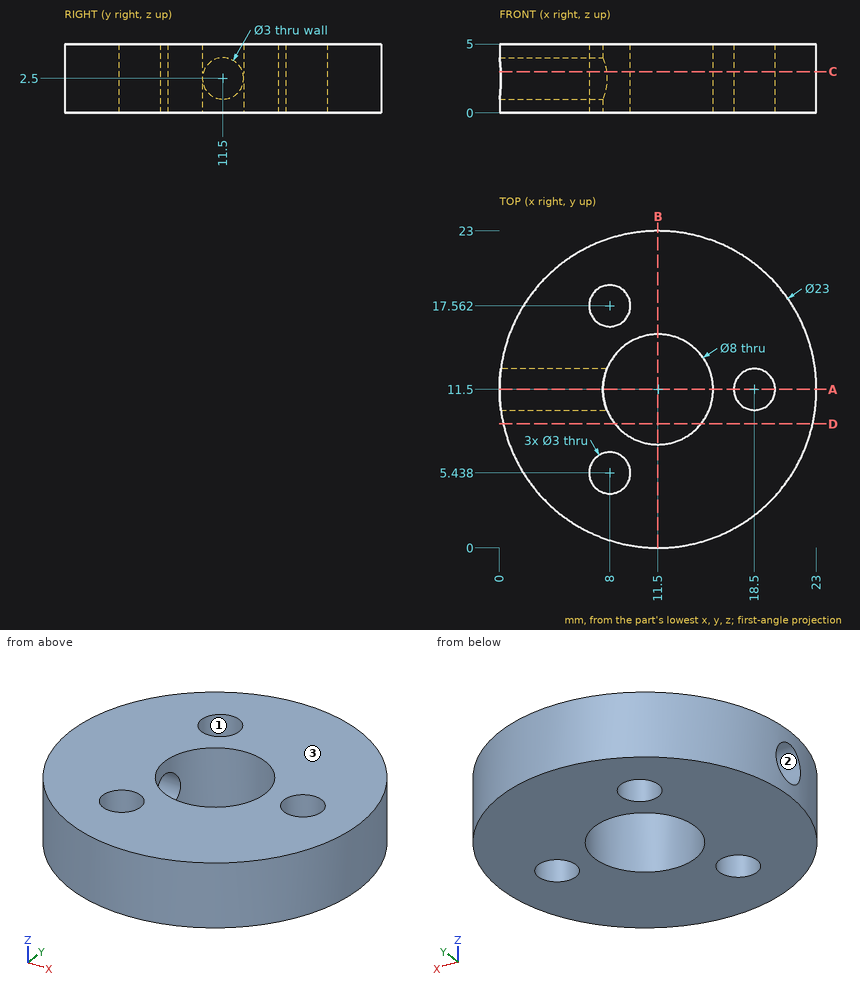
Input: dimensioned drawing with shaded views. Units: mm. Origin: part minimum x, y, z. Round coordinates to 2 decimals unless told otherwise and drop trailing zeros. Loops run counter-clockwise (first coordinate to the right, second up) from the corner with the lowest first, then second, coordinate; pieces in that order, holes last. Notation, with made-up numbers: M 68,-19 L 80,-19 A4 ccw 80,-12 Z; hole C 20,71.25 d8. An arc over 180 degrees is marked long. Answer in a Markdown table with one row per item. Add a question column.
1. Section C-C (z = 3). Output: boundary loops of the cut face in (x, y), and give its area (3 significant figures).
2. Mould query, pull axis Z, two halves, no side actions, for the marked faces 1, 2 and 3. Classes: released by +Z, released by -Z, zero draft, split by the parting line, or undercut.
3. Contact query for flat-ended pins moving along their axis: pin 1 (8 mm diameter, centred on x = 9, y = 9.5, fed in from -Z); pin 2 (1 mm diameter, centred on x = 4.5, z = 4, fed in from -Y); pin 3 (1 mm diameter, centred on x = 13, z = 1.5, fed in from -Y). Output: stop coordinate, or through.
4. Section A-A (y = 11.5). Output: boundary loops of the cut face in (x, z), and give its area (3 significant figures).
5. Ray query, probe 1 along Y at (x, z) = (8, 3.2) (1 decimal); probe 2 along Y at (x, z) = (11.5, 4.55); probe 3 along Y at (x, z) = (19, 2.5) (1 decimal). Return the intervals inside material, ascending.
6. Section D-D (y = 9). Output: boundary loops of the cut face in (x, z) (1 decimal).
7. Section B-B (x = 11.5). Output: boundary loops of the cut face in (y, z), and give its area (3 significant figures).
Values follow:
| question | item | result |
|---|---|---|
| 1 | outline | M 0.09,10.09 A11.5 ccw long 0.09,12.91 L 7.76,12.91 A4 cw long 7.76,10.09 Z; hole C 8,5.44 d3; hole C 8,17.56 d3; hole C 18.5,11.5 d3 |
| 1 | area | 323 mm^2 |
| 2 | face 1 | zero draft |
| 2 | face 2 | undercut |
| 2 | face 3 | released by +Z |
| 3 | pin 1 | z = 0 |
| 3 | pin 2 | y = 2.01 |
| 3 | pin 3 | y = 0.04 |
| 4 | outline | M 0,0 L 7.5,0 L 7.5,1 L 0,1 Z; M 0,4 L 7.5,4 L 7.5,5 L 0,5 Z; M 15.5,0 L 17,0 L 17,5 L 15.5,5 Z; M 20,0 L 23,0 L 23,5 L 20,5 Z |
| 4 | area | 37.5 mm^2 |
| 5 | probe 1 | 0.5 to 3.9, 6.9 to 9.6, 13.4 to 16.1, 19.1 to 22.5 |
| 5 | probe 2 | 0 to 7.5, 15.5 to 23 |
| 5 | probe 3 | 2.8 to 10.1, 12.9 to 20.2 |
| 6 | outline | M 0.3,0 L 8.4,0 L 8.4,5 L 0.3,5 Z; M 14.6,0 L 22.7,0 L 22.7,5 L 14.6,5 Z |
| 7 | outline | M 0,0 L 7.5,0 L 7.5,5 L 0,5 Z; M 15.5,0 L 23,0 L 23,5 L 15.5,5 Z |
| 7 | area | 75.0 mm^2 |
